Work out the finished part from the listing and answer in its coordinate system (mm). Face numbers are marked on the shaded views. Coordinates: 2 decimals unless noted, no trailing zeros. Order: outer loops, then holes, each group sorted by start corner. A loop starts at its lowest first (then second) coordinate and runs counter-clockwise, first axis right, second up. Notation, with made-up numbers: M 31,-12 L 37,-12 A32 ccw 37,27 Z; hole C 1.25,63.25 d11. An arc over 180 degrees is marked long. Use a Markdown table: item, result.
from build123d import *

# Parameters (mm, degrees)
EXTRUDE_1_DEPTH    = 8
HOLE_WIZARD_M161_D = 14
CHAMFER_1_SIZE     = 1.5


with BuildPart() as part:
    # Эскиз1 → Бобышка-Вытянуть1 (new body)
    with BuildSketch(Plane.XY):
        Polygon((0, 13.856406461), (-12, 6.92820323), (-12, -6.92820323), (0, -13.856406461), (12, -6.92820323), (12, 6.92820323), align=None)
    extrude(amount=EXTRUDE_1_DEPTH)

    # Отверстие обработанное метчиком M161 (through all)
    with Locations(Plane(origin=(0, 0, 0), x_dir=(-1, 0, 0), z_dir=(0, 0, -1))):
        with Locations((0, 0)):
            Hole(HOLE_WIZARD_M161_D / 2)

    # Фаска1
    chamfer_1_edges = [part.edges().sort_by_distance(p)[0] for p in [
        (-7, 0, 0),
        (-7, 0, 8),
    ]]
    chamfer(chamfer_1_edges, length=CHAMFER_1_SIZE)


solid = part.part
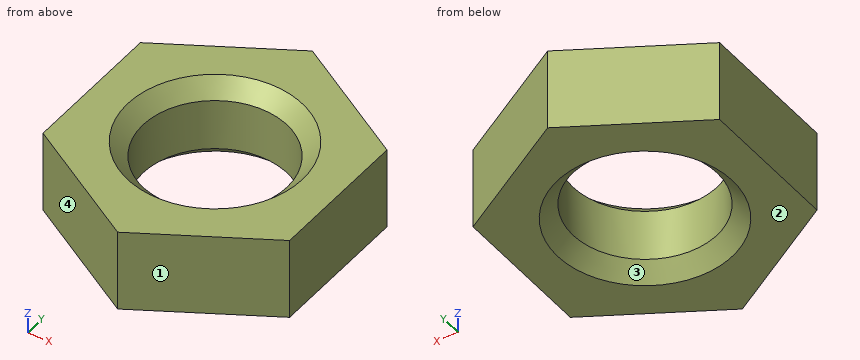
1. Section C-C on z = 4.25 is taken. Determine the outline of the cut face in (x, y), then the cut area to 3 significant figures.
Answers below:
| item | result |
|---|---|
| outline | M -12,-6.93 L 0,-13.86 L 12,-6.93 L 12,6.93 L 0,13.86 L -12,6.93 Z; hole C 0,0 d14 |
| area | 345 mm² |
2. Flat-ended cylindrical pins translate along their axes: P1, Ø4, axis at x = -4.5, z = 5.5, coming from the +Y side; P2, Ø1, axis at x = 1.5, z = 2.5, coming from the +Y side; P3, Ø3, axis at y = -9.5, z = 5, coming from the -X side; P4, Ø11, axis at x = 0, y = 0, coming from the +Z side. Find the tip coordinate at first contact, or state that the pin passes through.
Answers below:
| item | result |
|---|---|
| P1 | y = 12.41 |
| P2 | y = 13.28 |
| P3 | x = -10.14 |
| P4 | through |
3. Find the intervals of material crossed by probe 1 along Y at (x, z) = (4, 7.25); probe 2 along Y at (x, z) = (1.25, 5.5); probe 3 along X at (y, z) = (4, 7), in increasing order.
Answers below:
| item | result |
|---|---|
| probe 1 | -11.55 to -6.64, 6.64 to 11.55 |
| probe 2 | -13.13 to -6.89, 6.89 to 13.13 |
| probe 3 | -12 to -6.34, 6.34 to 12 |
4. Section B-B on z = 1 is taken. Determine the outline of the cut face in (x, y), then the cut area to 3 significant figures.
Answers below:
| item | result |
|---|---|
| outline | M -12,-6.93 L 0,-13.86 L 12,-6.93 L 12,6.93 L 0,13.86 L -12,6.93 Z; hole C 0,0 d15 |
| area | 322 mm² |
5. For a pull along X with two mould halves and no side action, classify the marked faces 1, 2, 3 and 4 as +X half, -X half, draft (parallel to the pull), parting line (faces both ways), or undercut.
Answers below:
| item | result |
|---|---|
| face 1 | +X half |
| face 2 | draft |
| face 3 | undercut |
| face 4 | -X half |
6. Section D-D on x = 9.25 is taken. Determine the outline of the cut face in (y, z), then the cut area to 3 significant figures.
Answers below:
| item | result |
|---|---|
| outline | M -8.52,0 L 8.52,0 L 8.52,8 L -8.52,8 Z |
| area | 136 mm² |
7. Section A-A on y = 0 is taken. Determine the outline of the cut face in (x, z), then the cut area to 3 significant figures.
Answers below:
| item | result |
|---|---|
| outline | M -12,0 L -8.5,0 L -7,1.5 L -7,6.5 L -8.5,8 L -12,8 Z; M 7,1.5 L 8.5,0 L 12,0 L 12,8 L 8.5,8 L 7,6.5 Z |
| area | 75.5 mm² |
